Part print with two shaded views. Sizes in mm from the minimum x, y, z corner. Coordinates: 2 decimals unless noted, no trailing zeros. Write each loop counter-clockwise with the first axis right and the second up, starting at its lowest first coordinate (ties: lowest second). Pieces come first, ordered by that corner, then holes. Notation, with made-up numbers: (42.25, 17) - (99.25, 17) arc R23 ccw to (99.25, 53) - close; hole circle Ø4 at (-15.5, 70). An arc over 180 degrees is marked (long way). Answer in a Markdown table with one row per item. Add a question column.
Q1. Band-saw the part on C-C (z = 4.7). List the corners of the cut face in (x, y), and give its area (3 significant figures).
Q2. Drill centre lines: line 1 along Y through (x, z) = (11.05, 1.95); line 2 along Y through (x, z) = (11.05, 0.25); line 3 along X through (y, z) = (10.25, 3.35). Where is each one in solid material? Low to high. Write a range as from..to.
Q3. Pin check, flat tips, straight feed: pin 1 (10.5 mm diameter, centred on x = 6.5, y = 14.5, fed in from +Z); pin 2 (12.5 mm diameter, centred on x = 11.05, y = 11.05, fed in from -Z); pin 3 (1.5 mm diameter, centred on y = 15.5, z = 4.5, fed in from +X); pin 4 (1 mm diameter, centred on y = 14, z = 2, fed in from +X) (3 decimals). Stop position of each tip, or through.
Q4. Band-saw the part on A-A (y = 11.05). List the corners of the cut face in (x, z).
Q5. Two-plate mould, pull along Y, no slides. Class the marked faces 1, 2 and 3: +Y half, -Y half, draft (parallel to the pull), parting line (faces both ways), or undercut.
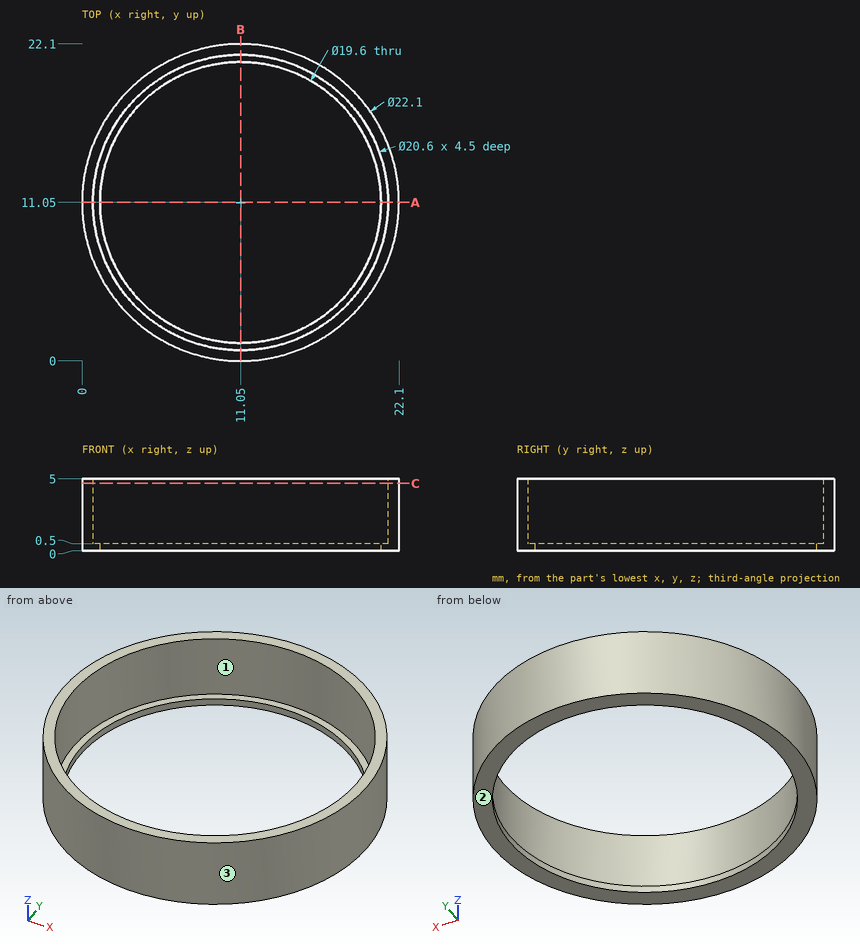
Checked values:
| question | item | result |
|---|---|---|
| 1 | outline | circle Ø22.1 at (11.05, 11.05); hole circle Ø20.6 at (11.05, 11.05) |
| 1 | area | 50.3 mm² |
| 2 | line 1 | y = 0..0.75, 21.35..22.1 |
| 2 | line 2 | y = 0..1.25, 20.85..22.1 |
| 2 | line 3 | x = 0.03..0.78, 21.32..22.07 |
| 3 | pin 1 | stops at z = 5 |
| 3 | pin 2 | passes through |
| 3 | pin 3 | stops at x = 21.46 |
| 3 | pin 4 | stops at x = 21.825 |
| 4 | outline | (0, 0) - (1.25, 0) - (1.25, 0.5) - (0.75, 0.5) - (0.75, 5) - (0, 5) - close; (20.85, 0) - (22.1, 0) - (22.1, 5) - (21.35, 5) - (21.35, 0.5) - (20.85, 0.5) - close |
| 5 | face 1 | undercut |
| 5 | face 2 | draft |
| 5 | face 3 | parting line |
